Input: part model. Units: mm. Frame: model coordinates. A direction names the side the tool comes from. Coordinates: 2 decimals unless noted, no trailing zeros. Use one line per item in the form item = value.
Autodesk Inventor part; units mm, degrees
ref_plane "YZ Plane" through (0, 0, 0) normal (1, 0, 0) x (0, 1, 0)
ref_plane "XZ Plane" through (0, 0, 0) normal (0, 1, 0) x (-1, 0, 0)
ref_plane "XY Plane" through (0, 0, 0) normal (0, 0, 1) x (1, 0, 0)
sketch "Sketch1" plane through (0, 0, 0) normal (1, 0, 0) x (0, 1, 0)
  circle A0 centre (0, 0) radius 14.75 construction
  line L0 (2.75, -1.5877) -> (0, -3.1754)
  line L1 (0, -3.1754) -> (-2.75, -1.5877)
  line L2 (-2.75, -1.5877) -> (-2.75, 1.5877)
  line L3 (-2.75, 1.5877) -> (0, 3.1754)
  line L4 (0, 3.1754) -> (2.75, 1.5877)
  line L5 (2.75, 1.5877) -> (2.75, -1.5877)
  line L6 (14.5684, 2.3074) -> (14.5684, -2.3074) construction
  line L7 (14.5684, 2.3074) -> (0, 0) construction
  line L8 (0, 0) -> (14.5684, -2.3074) construction
  line L9 (14.5684, 2.3074) -> (13.5684, 0)
  line L10 (13.5684, 0) -> (14.5684, -2.3074)
  line L11 (13.5684, 0) -> (14.5684, 0) construction
  line L12 (13.1423, 6.6964) -> (12.9043, 4.1929)
  line L13 (12.9043, 4.1929) -> (14.5684, 2.3074)
  line L14 (10.4298, 10.4298) -> (10.9771, 7.9753)
  line L15 (10.9771, 7.9753) -> (13.1423, 6.6964)
  line L16 (6.6964, 13.1423) -> (7.9753, 10.9771)
  line L17 (7.9753, 10.9771) -> (10.4298, 10.4298)
  line L18 (2.3074, 14.5684) -> (4.1929, 12.9043)
  line L19 (4.1929, 12.9043) -> (6.6964, 13.1423)
  line L20 (-2.3074, 14.5684) -> (0, 13.5684)
  line L21 (0, 13.5684) -> (2.3074, 14.5684)
  line L22 (-6.6964, 13.1423) -> (-4.1929, 12.9043)
  line L23 (-4.1929, 12.9043) -> (-2.3074, 14.5684)
  line L24 (-10.4298, 10.4298) -> (-7.9753, 10.9771)
  line L25 (-7.9753, 10.9771) -> (-6.6964, 13.1423)
  line L26 (-13.1423, 6.6964) -> (-10.9771, 7.9753)
  line L27 (-10.9771, 7.9753) -> (-10.4298, 10.4298)
  line L28 (-14.5684, 2.3074) -> (-12.9043, 4.1929)
  line L29 (-12.9043, 4.1929) -> (-13.1423, 6.6964)
  line L30 (-14.5684, -2.3074) -> (-13.5684, 0)
  line L31 (-13.5684, 0) -> (-14.5684, 2.3074)
  line L32 (-13.1423, -6.6964) -> (-12.9043, -4.1929)
  line L33 (-12.9043, -4.1929) -> (-14.5684, -2.3074)
  line L34 (-10.4298, -10.4298) -> (-10.9771, -7.9753)
  line L35 (-10.9771, -7.9753) -> (-13.1423, -6.6964)
  line L36 (-6.6964, -13.1423) -> (-7.9753, -10.9771)
  line L37 (-7.9753, -10.9771) -> (-10.4298, -10.4298)
  line L38 (-2.3074, -14.5684) -> (-4.1929, -12.9043)
  line L39 (-4.1929, -12.9043) -> (-6.6964, -13.1423)
  line L40 (2.3074, -14.5684) -> (0, -13.5684)
  line L41 (0, -13.5684) -> (-2.3074, -14.5684)
  line L42 (6.6964, -13.1423) -> (4.1929, -12.9043)
  line L43 (4.1929, -12.9043) -> (2.3074, -14.5684)
  line L44 (10.4298, -10.4298) -> (7.9753, -10.9771)
  line L45 (7.9753, -10.9771) -> (6.6964, -13.1423)
  line L46 (13.1423, -6.6964) -> (10.9771, -7.9753)
  line L47 (10.9771, -7.9753) -> (10.4298, -10.4298)
  line L48 (14.5684, -2.3074) -> (12.9043, -4.1929)
  line L49 (12.9043, -4.1929) -> (13.1423, -6.6964)
  dimension "d0" = 29.5
  dimension "d1" = 5.5
  dimension "d2" = 18
  dimension "d3" = 1
  dimension "d6" = 360
extrude "Extrusion1" add sketch "Sketch1" along normal mid plane 70
sketch "Sketch2" plane through (0, 0, 0) normal (0, 0, 1) x (1, 0, 0)
  line L0 (-35, 14.5684) -> (35, 14.5684)
  line L1 (-35, -14.5684) -> (35, -14.5684)
  line L2 (-35, 14.5684) -> (-25, 14.5684)
  line L3 (-25, 14.5684) -> (-25, -14.5684)
  line L4 (-25, -14.5684) -> (-35, -14.5684)
  line L5 (-35, -14.5684) -> (-35, 14.5684)
  line L6 (-35, 4.5684) -> (-25, 4.5684)
  line L7 (-35, 14.5684) -> (-35, 14.5684)
  line L8 (-35, 14.5684) -> (-33, 14.5684)
  line L9 (-25, 14.5684) -> (-25, 14.5684)
  line L10 (-25, 14.5684) -> (-27, 14.5684)
  arc A0 (-33, 14.5684) -> (-27, 14.5684) centre (-30, 16.3712) ccw
  line L11 (-35, 0) -> (35, 0)
  line L12 (-35, 0) -> (-25, 0)
  line L13 (-35, 14.5684) -> (-25, 14.5684)
  line L14 (-25, 14.5684) -> (-25, 20.6242)
  line L15 (-25, 20.6242) -> (-35, 20.6242)
  line L16 (-35, 20.6242) -> (-35, 14.5684)
  point P0 (0, 0)
  dimension "d11" = 0
  dimension "d12" = 10
  dimension "d13" = 10
  dimension "d14" = 2
  dimension "d15" = 0
  dimension "d16" = 2
  dimension "d17" = 0
  dimension "d18" = 3.5
revolve "Revolution2" cut sketch "Sketch2" angle 360 about axis through (-35, 0, 0) along (1, 0, 0) contours L16 L15 L14 L0 | L0 A0 L3 L6 L5 | L0 A0
revolve "Revolution1" add sketch "Sketch2" angle 360 about axis through (-35, 0, 0) along (1, 0, 0) contours L0 A0 L3 L6 L5
properties part number "SolidRoller" material "PC/ABS Plastic"
(1) Set-up query: faces 5 (the flat face through (5, -14, 1)), 6 (the flat face through (4.58, 9.185, 10.707)), 7 (the flat face through (-25, 13.5, -4.4)), 8 (the flat face through (4.58, -10.707, 9.185)), 9 (the flat face through (-0.49, -1.394, 2.37)). Return all of +Z, -Z, +X, -X, +Y, -Y with unobstructed straight access to the full face (end or side cutting, diameter ignored); none if empty.
Computed:
face_5 = +X, -Y
face_6 = +Z, +X, +Y
face_7 = +X, +Y
face_8 = +Z, +X, -Y
face_9 = +X, -X
(2) Pull-direction query (Y, two-part tool) for faces 1 (the flat face through (0, -2.75, 0)), 2 (the flat face through (4.58, 10.7, 9.22)), 3 (the flat face through (4.58, -5.462, 13.025)), 4 (the flat face through (-25, 11.5, -8.4)); classes: pulls with the +Y half, pulls with the -Y half, needs draft (parallel to the pull), parting line crosses it, or undercut.
Computed:
face_1 = undercut
face_2 = pulls with the +Y half
face_3 = undercut
face_4 = needs draft
(3) Line query: probe 1 along Y at (x, z) = (5, 0); probe 2 along Z at (x, y) = (-28.5, 8.5); probe 3 along Y at (x, z) = (-26, -1.25). Output: solid intervals per line, ascending.
Computed:
probe_1 = -13.57 to -2.75, 2.75 to 13.57
probe_2 = -10.11 to 10.11
probe_3 = -14.51 to -2.75, 2.75 to 14.51
(4) First-contact query: pin 1 Ø2.5 at (y, z) = (8.5, -12) entering from +X; pin 2 Ø1.5 at (x, z) = (7.5, 6.5) entering from -Y; pin 3 Ø3 at (x, y) = (-21.5, -5.5) entering from -Z; pin 4 Ø5 at (x, y) = (21.5, 10) entering from +Z. Flat tips, straight axial feed; report the tip coordinate or a pass-through.
Computed:
pin_1 = 35
pin_2 = -13.14
pin_3 = -13.14
pin_4 = 11.78
